from build123d import *

# Parameters (mm, degrees)
EXTRUDE_1_DEPTH         = 3.2
SKETCH_4_R              = 16
CUT_EXTRUDE_1_DEPTH     = 6
HOLE_WIZARD_3_1_3_1_4_D = 3.1


with BuildPart() as part:
    # Эскиз1 → Бобышка-Вытянуть1 (new body)
    with BuildSketch(Plane.XY):
        Polygon((50, -3.2), (-50, -3.2), (-50, -53.2), (-60, -53.2), (-80, 45), (-80, 115), (-60, 213.2), (-50, 213.2), (-50, 163.2), (50, 163.2), (50, 213.2), (70, 213.2), (190, 105), (190, 55), (70, -53.2), (50, -53.2), align=None)
    extrude(amount=EXTRUDE_1_DEPTH)

    # Эскиз4 → Вырез-Вытянуть1 (cut)
    with BuildSketch(Plane.XY.offset(3.2)):
        with Locations((155.25, 79.5275375)):
            Circle(SKETCH_4_R)
    extrude(amount=-CUT_EXTRUDE_1_DEPTH, mode=Mode.SUBTRACT)

    # Диаметр отверстия Ø3.1 (3.1)4 (through all)
    with Locations(Plane(origin=(0, 0, 0), x_dir=(-1, 0, 0), z_dir=(0, 0, -1))):
        with Locations((-145.85, 95.808815091), (-145.85, 63.246259909), (-174.05, 79.5275375)):
            Hole(HOLE_WIZARD_3_1_3_1_4_D / 2)


solid = part.part
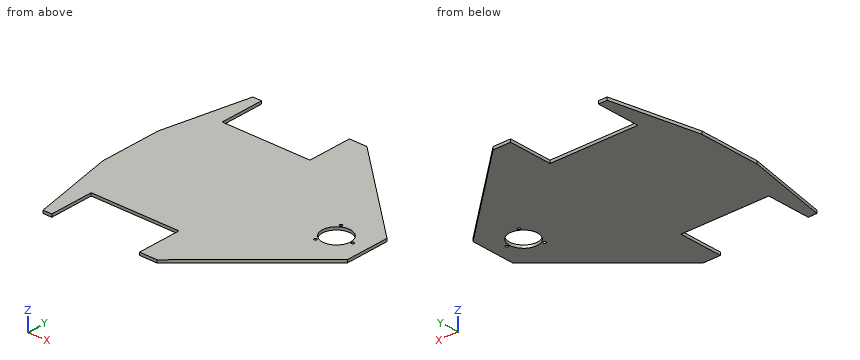
Geometry check sheet. Reference: the model listing, model coordinates, mm. Give positions to 0.01 mm unless a question says otherwise; leave off trailing zeros. Write each loop counter-clockwise with the first axis right and the second up, starting at its lowest first coordinate (ties: lowest second). Pieces come first, ordered by that corner, then holes.
1) Cross-section at B-B (z = 1.7). Record the boundary of the cut face in (x, y), plus the area to 3 significant figures.
Values follow:
outline: (-80, 45) - (-60, -53.2) - (-50, -53.2) - (-50, -3.2) - (50, -3.2) - (50, -53.2) - (70, -53.2) - (190, 55) - (190, 105) - (70, 213.2) - (50, 213.2) - (50, 163.2) - (-50, 163.2) - (-50, 213.2) - (-60, 213.2) - (-80, 115) - close; hole circle Ø32 at (155.25, 79.53); hole circle Ø3.1 at (145.85, 63.25); hole circle Ø3.1 at (145.85, 95.81); hole circle Ø3.1 at (174.05, 79.53)
area: 46,200 mm2
2) Cross-section at A-A (y = 184). Record the boundary of the cut face in (x, z), plus the area to 3 significant figures.
Values follow:
outline: (-65.95, 0) - (-50, 0) - (-50, 3.2) - (-65.95, 3.2) - close; (50, 0) - (102.38, 0) - (102.38, 3.2) - (50, 3.2) - close
area: 219 mm2
3) Cross-section at C-C (x = 155.25). Record the boundary of the cut face in (y, z), plus the area to 3 significant figures.
Values follow:
outline: (23.67, 0) - (63.53, 0) - (63.53, 3.2) - (23.67, 3.2) - close; (95.53, 0) - (136.33, 0) - (136.33, 3.2) - (95.53, 3.2) - close
area: 258 mm2
4) Thickness scan on line 1 (Y direction, x = 145.85, z = 1.4); line 2 (Y direction, x = 15, z = 0.2); line 3 (X direction, y = 149, z = 2.25). Record the ranges inside material, lowest first.
Values follow:
line 1: y = 15.19 to 61.7, 64.8 to 66.58, 92.48 to 94.26, 97.36 to 144.81
line 2: y = -3.2 to 163.2
line 3: x = -73.08 to 141.2
5) Cross-section at D-D (x = 84.5). Record the boundary of the cut face in (y, z), plus the area to 3 significant figures.
Values follow:
outline: (-40.13, 0) - (200.13, 0) - (200.13, 3.2) - (-40.13, 3.2) - close
area: 769 mm2
6) Go/stop test with flat-tipped pins: pin 1 Ø1.6 at (x, z) = (-3, 1) entering from +Y; pin 2 Ø1.6 at (y, z) = (-33, 2) entering from +X; pin 3 Ø1.6 at (y, z) = (181.5, 1.5) entering from -X; pin 4 Ø3.5 at (x, y) = (145.85, 95.81) entering from +Z. Record where each tip stops, or that it passes through.
Values follow:
pin 1: stops at y = 163.2
pin 2: stops at x = 93.29
pin 3: stops at x = -66.62
pin 4: stops at z = 3.2
